from build123d import *

# Parameters (mm, degrees)
SKETCH2_R           = 3.048
BOSS_EXTRUDE1_DEPTH = 5.07492
CUT_EXTRUDE11_DEPTH = 210.646067011
SKETCH3_R           = 6.35
SKETCH3_R_2         = 2.032
CUT_EXTRUDE12_DEPTH = 210.646067011
SKETCH5_R           = 1.4732
CUT_EXTRUDE13_DEPTH = 210.646067011
SKETCH7_R           = 1.905
CUT_EXTRUDE14_DEPTH = 210.646067011
SKETCH9_R           = 2.794
CUT_EXTRUDE16_DEPTH = 5.08


with BuildPart() as part:
    # Sketch2 → Boss-Extrude1 (new body)
    with BuildSketch(Plane.XY):
        with BuildLine():
            Line((-186.69, -31.75), (-144.826640797, -31.75))
            ThreePointArc((-144.826640797, -31.75), (-123.19, -59.055), (-101.553359203, -31.75))
            Line((-101.553359203, -31.75), (101.553359203, -31.75))
            ThreePointArc((101.553359203, -31.75), (123.19, -59.055), (144.826640797, -31.75))
            Line((144.826640797, -31.75), (186.69, -31.75))
            Line((186.69, -31.75), (186.69, 95.25))
            Line((186.69, 95.25), (-186.69, 95.25))
            Line((-186.69, 95.25), (-186.69, -31.75))
        make_face()
        with Locations((-86.868, -16.51)):
            Circle(SKETCH2_R, mode=Mode.SUBTRACT)
        with Locations((86.868, -16.51)):
            Circle(SKETCH2_R, mode=Mode.SUBTRACT)
        with Locations((123.19, 76.2)):
            Circle(SKETCH2_R, mode=Mode.SUBTRACT)
        with Locations((-123.19, 76.2)):
            Circle(SKETCH2_R, mode=Mode.SUBTRACT)
    extrude(amount=-BOSS_EXTRUDE1_DEPTH)

    # Sketch2_4 → Cut-Extrude11 (cut, through all)
    with BuildSketch(Plane.XY):
        with BuildLine():
            ThreePointArc((-119.486801079, -31.75), (-123.19, -30.5435), (-126.893198921, -31.75))
            Line((-126.893198921, -31.75), (-119.486801079, -31.75))
        make_face()
        with BuildLine():
            Line((-119.486801079, -31.75), (-126.893198921, -31.75))
            ThreePointArc((-126.893198921, -31.75), (-126.039554547, -42.433581099), (-116.9035, -36.83))
            ThreePointArc((-116.9035, -36.83), (-117.586418901, -33.980445453), (-119.486801079, -31.75))
        make_face()
        with BuildLine():
            ThreePointArc((126.893198921, -31.75), (123.19, -30.5435), (119.486801079, -31.75))
            Line((119.486801079, -31.75), (126.893198921, -31.75))
        make_face()
        with BuildLine():
            Line((126.893198921, -31.75), (119.486801079, -31.75))
            ThreePointArc((119.486801079, -31.75), (120.340445453, -42.433581099), (129.4765, -36.83))
            ThreePointArc((129.4765, -36.83), (128.793581099, -33.980445453), (126.893198921, -31.75))
        make_face()
    extrude(amount=-CUT_EXTRUDE11_DEPTH, mode=Mode.SUBTRACT)

    # Sketch3 → Cut-Extrude12 (cut, through all)
    with BuildSketch(Plane.XY):
        with Locations((-9.090770625, 1.27)):
            Circle(SKETCH3_R)
        with Locations((8.435229375, 1.27)):
            Circle(SKETCH3_R_2)
        with Locations((54.450542101, 51.954711472)):
            Circle(SKETCH3_R)
        with Locations((71.976542101, 51.954711472)):
            Circle(SKETCH3_R_2)
        with Locations((54.450542101, 69.480711472)):
            Circle(SKETCH3_R_2)
        with Locations((36.924542101, 51.954711472)):
            Circle(SKETCH3_R_2)
        with Locations((-9.090770625, 18.796)):
            Circle(SKETCH3_R_2)
        with Locations((-26.616770625, 1.27)):
            Circle(SKETCH3_R_2)
        with Locations((-9.090770625, -16.256)):
            Circle(SKETCH3_R_2)
        with Locations((54.450542101, 34.428711472)):
            Circle(SKETCH3_R_2)
    extrude(amount=-CUT_EXTRUDE12_DEPTH, mode=Mode.SUBTRACT)

    # Sketch5 → Cut-Extrude13 (cut, through all)
    with BuildSketch(Plane.XY):
        with Locations((-29.227921948, -21.947964868)):
            Circle(SKETCH5_R)
        with Locations((11.046380698, -21.947964868)):
            Circle(SKETCH5_R)
        with Locations((-39.274550202, -4.519491037)):
            Circle(SKETCH5_R)
        with Locations((21.093008951, -4.519491037)):
            Circle(SKETCH5_R)
        with Locations((34.313390778, 28.736746605)):
            Circle(SKETCH5_R)
        with Locations((74.587693424, 28.736746605)):
            Circle(SKETCH5_R)
        with Locations((24.266762524, 46.165220436)):
            Circle(SKETCH5_R)
        with Locations((84.634321678, 46.165220436)):
            Circle(SKETCH5_R)
    extrude(amount=-CUT_EXTRUDE13_DEPTH, mode=Mode.SUBTRACT)

    # Sketch7 → Cut-Extrude14 (cut, through all)
    with BuildSketch(Plane.XY):
        with Locations((131.572, -19.05)):
            Circle(SKETCH7_R)
        with Locations((114.808, -19.05)):
            Circle(SKETCH7_R)
        with Locations((-123.19, -49.022)):
            Circle(SKETCH7_R)
        with Locations((-131.572, -19.05)):
            Circle(SKETCH7_R)
        with Locations((-114.808, -19.05)):
            Circle(SKETCH7_R)
        with Locations((123.19, -49.022)):
            Circle(SKETCH7_R)
    extrude(amount=-CUT_EXTRUDE14_DEPTH, mode=Mode.SUBTRACT)

    # Sketch9 → Cut-Extrude16 (cut)
    with BuildSketch(Plane.XY):
        with Locations((55.88, -23.114)):
            Circle(SKETCH9_R)
    extrude(amount=-CUT_EXTRUDE16_DEPTH, mode=Mode.SUBTRACT)


solid = part.part
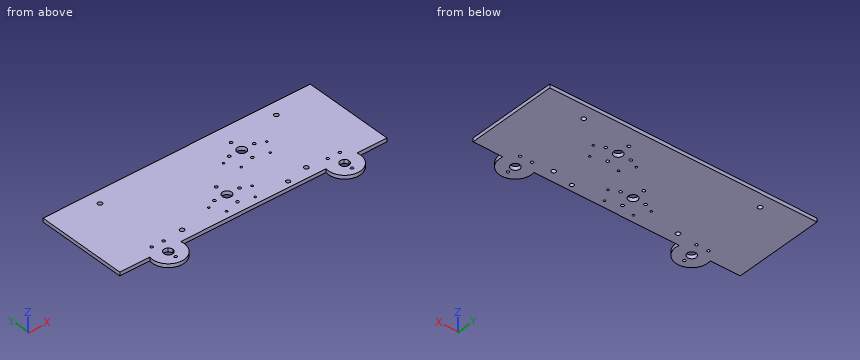
Work out the finished part from the listing and answer in its coordinate system (mm). Give positions to 0.01 mm unless a question says otherwise; leave off trailing zeros. Order: outer loops, then holes, each group sorted by start corner. A loop starts at its lowest first (then second) coordinate and runs counter-clockwise, first axis right, second up. Notation, with made-up numbers: (37.5, 11.5) -> (61.5, 11.5) arc R9 cw to (61.5, 19.5) -> close; hole circle Ø7 at (86.5, -2.5). An arc over 180 degrees is marked (long way). One line per item, written item: value.
Item 1: Find section A-A, the plane z = -1.15. State how many separate pieces and enclosed holes the cut face has, plus the area to 3 significant figures.
Answer sheet:
separate pieces: 1
enclosed holes: 31
area: 48,500 mm²
Item 2: Straight lines are drawn through the part: probe 1 along Y at (x, z) = (21.5, -1.3); probe 2 along X at (y, z) = (45, -4.15); probe 3 along X at (y, z) = (-20, -0.2). For each, find the intervals that lie inside material, in ascending order.
Answer sheet:
probe 1: -31.75 to -5.94, -3.1 to 95.25
probe 2: -186.69 to 23.37, 25.17 to 83.73, 85.54 to 186.69
probe 3: -186.69 to -133.22, -129.92 to -116.46, -113.16 to 113.16, 116.46 to 129.92, 133.22 to 186.69
Item 3: Flat-ended cylindrical pins translate along their axes: P1, Ø20.5, axis at x = 54.45, y = 51.95, coming from the -Z side; P2, Ø3.5, axis at x = 54.45, y = 34.43, coming from the +Z side. Find the tip coordinate at first contact, or state that the pin passes through.
Answer sheet:
P1: z = -5.07
P2: through
Item 4: Find section B-B, the plane x = -65.5. Give the vertices of the cut face in (y, z), plus the area to 3 significant figures.
Answer sheet:
outline: (-31.75, -5.07) -> (95.25, -5.07) -> (95.25, 0) -> (-31.75, 0) -> close
area: 645 mm²
